Can you work these out from the model? Positions are in its coordinate system, mm. A direction names the side the tool comes from. Give positions to 0.01 mm unless a question says otherwise; leave off trailing zeros. Loops run counter-clockwise (first coordinate to the right, second up) from the corner with the lowest first, then second, coordinate; pieces in that order, holes last. Notation, with made-up numbers: (42, -14.75) - (83, -14.75) arc R14 ccw to (83, 0.25) - close; hole circle Ø11 at (53, -36). An arc over 180 degrees is marked (long way). Answer as a JSON object with one key per item and string values.
```python
from build123d import *

# Parameters (mm, degrees)
SKETCH_W        = 200
SKETCH_H        = 70
PAD_DEPTH       = 33
SKETCH001_W     = 194
SKETCH001_H     = 67
POCKET_DEPTH    = 30
SKETCH002_W     = 169
SKETCH002_H     = 3
PAD001_DEPTH    = 23
SKETCH004_R     = 7.5
POCKET001_DEPTH = 5


with BuildPart() as part:
    # Sketch → Pad (new body)
    with BuildSketch(Plane.XY):
        Rectangle(SKETCH_W, SKETCH_H)
    extrude(amount=PAD_DEPTH)

    # Sketch001 (on Face6 of Pad) → Pocket (cut)
    with BuildSketch(Plane.XY.offset(33)):
        with Locations((0, -1.5)):
            Rectangle(SKETCH001_W, SKETCH001_H)
    extrude(amount=-POCKET_DEPTH, mode=Mode.SUBTRACT)

    # Sketch002 → Pad001 (join)
    with BuildSketch(Plane.XY):
        with Locations((0, -33.5)):
            Rectangle(SKETCH002_W, SKETCH002_H)
    extrude(amount=-PAD001_DEPTH)

    # Sketch004 (on Face14 of Pad001) → Pocket001 (cut)
    with BuildSketch(Plane.XZ.offset(35)):
        with Locations((0, -11.5)):
            Circle(SKETCH004_R)
        with Locations((-23, -11.5)):
            Circle(SKETCH004_R)
        with Locations((23, -11.5)):
            Circle(SKETCH004_R)
        with Locations((46, -11.5)):
            Circle(SKETCH004_R)
        with Locations((69, -11.5)):
            Circle(SKETCH004_R)
        with Locations((-46, -11.5)):
            Circle(SKETCH004_R)
        with Locations((-69, -11.5)):
            Circle(SKETCH004_R)
    extrude(amount=-POCKET001_DEPTH, mode=Mode.SUBTRACT)


solid = part.part
```
1) Imagine slicing it at C-C on y = 13.5. Write out the boundary of the cut face in (x, z).
Check sheet entries:
{"outline": "(-100, 0) - (100, 0) - (100, 33) - (97, 33) - (97, 3) - (-97, 3) - (-97, 33) - (-100, 33) - close"}
2) I'm going to push flat-ended pins straight in: P1, Ø13.5, axis at x = -46, z = -11.5, coming from the -Y side; P2, Ø6, axis at x = -36.5, y = -14.5, coming from the +Z side; P3, Ø1.5, axis at y = -33, z = -13.5, coming from the -X side; P4, Ø9, axis at x = 3, z = 10.5, coming from the -Y side. Where does each tip first touch, or does it pass through?
Check sheet entries:
{"P1": "through", "P2": "z = 3", "P3": "x = -84.5", "P4": "y = 32"}
3) Imagine slicing it at A-A on z = -11.5. Give the number of separate pieces and of enclosed holes in the cut face, and give its area (3 significant figures).
Check sheet entries:
{"separate pieces": "8", "enclosed holes": "0", "area": "192 mm2"}
4) Imagine slicing it at D-D on z = 12. Write out the boundary of the cut face in (x, y).
Check sheet entries:
{"outline": "(-100, -35) - (-97, -35) - (-97, 32) - (97, 32) - (97, -35) - (100, -35) - (100, 35) - (-100, 35) - close"}
5) Which directions (+Z, -Z, +X, -X, +Y, -Y) give clear straight access to the entire face, cutting with the end or side of a thin tool? Please do faces 4 (the cylindrical face through (61.507, -33.521, -11.17)), 5 (the flat face through (-97, -2, 18)), 6 (the flat face through (-1.2, -32, -3.7)).
Check sheet entries:
{"face 4": "+Y, -Y", "face 5": "+Z, -Y", "face 6": "-Z, +X, -X, +Y"}
6) I need wall thicknesses on L1, parallel to X at y = 5, z = 29; L2, parallel to Z at x = 23, y = -33.5; L3, parallel to Y at x = 29, z = 19. Which ranges of each line are inside material? Lowest first, please.
Check sheet entries:
{"L1": "-100 to -97, 97 to 100", "L2": "-23 to -19, -4 to 3", "L3": "32 to 35"}
7) If we mould it in two halves opening along X, with no side actions, what happens to faces 1 (the flat face through (-1, 0, 0)), 2 (the cylindrical face through (53.154, -33.521, -9.247)), 3 (the flat face through (-100, 0, 16))? For each: released by +X, released by -X, zero draft, split by the parting line, or undercut.
Check sheet entries:
{"face 1": "zero draft", "face 2": "undercut", "face 3": "released by -X"}
8) Imagine slicing it at B-B on x = 46. Write out the boundary of the cut face in (y, z), and give its area (3 significant figures).
Check sheet entries:
{"outline": "(-35, -23) - (-32, -23) - (-32, -19) - (-35, -19) - close; (-35, -4) - (-32, -4) - (-32, 0) - (35, 0) - (35, 33) - (32, 33) - (32, 3) - (-35, 3) - close", "area": "324 mm2"}
